Geometry: final body of the model. Coordinates: model frame, mm. Face numbers are marked on the shaded views. A direction names the side the tool comes from. Coordinates: 2 decimals unless noted, no trailing zeros. Loops run counter-clockwise (first coordinate to the right, second up) from the corner with the lowest first, then second, coordinate; pieces in that order, holes last. Notation, with made-up numbers: (69, 77.25) - (80, 77.25) arc R20 cw to (80, 115.25) - close; hole circle Ø11 at (-0.5, 11.25). An arc over 180 degrees is marked (long way). Put each result on its own line as item: value. Start each with the question number.
1) Section A-A on x = 0. Output: boundary loops of the cut face in (y, z).
2) Draft query along Y for the marked faces 1, 2 and 3. Return one class per face: +Y half, -Y half, draft (parallel to the pull), parting line (faces both ways), or undercut.
3) Reachability of the marked faces 4 and 5 from +Z, -Z, +X, -X, +Y, -Y: full face, straight path, thin tool, end or side. Return the list, or none.
4) Material intervals for line 1 along Z through (x, y) = (-1.5, -2); line 2 along Y through (x, z) = (0, 4.75); line 3 along Y through (x, z) = (0.25, 3.25), sorted ascending. Write a range as from..to.
5) Section C-C on z = 4.5. Output: boundary loops of the cut face in (x, y).
6) Contact query for flat-ended pins moving along their axis: pin 1 Ø0.9 at (y, z) = (0, 3) entering from +X; pin 2 Ø1.8 at (x, y) = (0, 0) entering from -Z (3 decimals). Output: stop coordinate, or through.
7) Section B-B on y = 0. Output: boundary loops of the cut face in (x, z), and give its area (3 significant figures).
8) Section D-D on y = 1.75. Output: boundary loops of the cut face in (x, z), and give its area (3 significant figures).
```python
from build123d import *

# Parameters (mm, degrees)
BOX009_W     = 8.5
BOX009_H     = 8
BOX009_DEPTH = 3
SKETCH013_W  = 8.045495
SKETCH013_H  = 10.974572
SKETCH013_R  = 1.530969
PAD013_DEPTH = 5


with BuildPart() as body059:
    # Box009 → Box009 (new body)
    with BuildSketch(Plane(origin=(-3, -4, 1), x_dir=(1, 0, 0), z_dir=(0, 0, 1))):
        with Locations((4.25, 4)):
            Rectangle(BOX009_W, BOX009_H)
    extrude(amount=BOX009_DEPTH)


with BuildPart() as body059_1:
    # BaseFeature015 placement: moved
    add(body059.part.moved(Location((3, 4, -1))))


with BuildPart() as body059_2:
    # Body059 placement: moved
    add(body059_1.part.moved(Location((-3, -4, 1))))


with BuildPart() as cut011:
    # Sketch013 → Pad013 (new body)
    with BuildSketch(Plane.XY):
        with Locations((1.022447, -0.012719)):
            Rectangle(SKETCH013_W, SKETCH013_H)
        Circle(SKETCH013_R, mode=Mode.SUBTRACT)
    extrude(amount=PAD013_DEPTH)

    # Cut011: cut Body059
    add(body059_2.part, mode=Mode.SUBTRACT)


solid = cut011.part
```
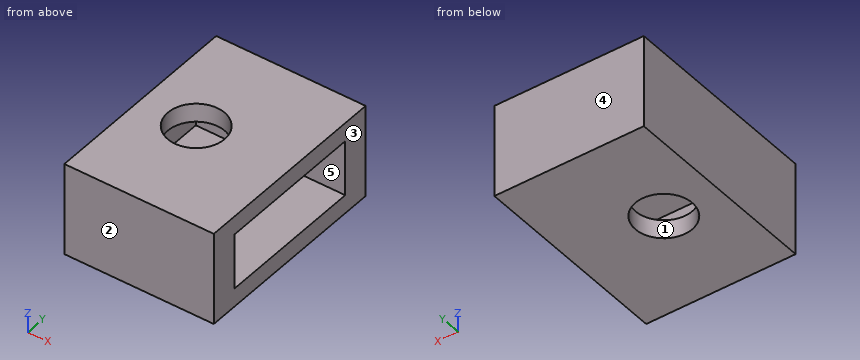
Answer block:
1. outline: (-5.5, 0) - (-1.53, 0) - (-1.53, 1) - (-4, 1) - (-4, 4) - (-1.53, 4) - (-1.53, 5) - (-5.5, 5) - close; (1.53, 0) - (5.47, 0) - (5.47, 5) - (1.53, 5) - (1.53, 4) - (4, 4) - (4, 1) - (1.53, 1) - close
2. face 1: undercut
2. face 2: -Y half
2. face 3: draft
3. face 4: +Z, -Z, +X, -X, +Y
3. face 5: +X
4. line 1: z = 0..1, 4..5
4. line 2: y = -5.5..-1.53, 1.53..5.47
4. line 3: y = -5.5..-4, 4..5.47
5. outline: (-3, -5.5) - (5.05, -5.5) - (5.05, 5.47) - (-3, 5.47) - close; hole circle Ø3.06 at (0, 0)
6. pin 1: stops at x = -3
6. pin 2: passes through
7. outline: (-3, 0) - (-1.53, 0) - (-1.53, 1) - (-3, 1) - (-3, 4) - (-1.53, 4) - (-1.53, 5) - (-3, 5) - close; (1.53, 0) - (5.05, 0) - (5.05, 1) - (1.53, 1) - close; (1.53, 4) - (5.05, 4) - (5.05, 5) - (1.53, 5) - close
7. area: 9.97 mm²
8. outline: (-3, 0) - (5.05, 0) - (5.05, 1) - (-3, 1) - (-3, 4) - (5.05, 4) - (5.05, 5) - (-3, 5) - close
8. area: 16.1 mm²
